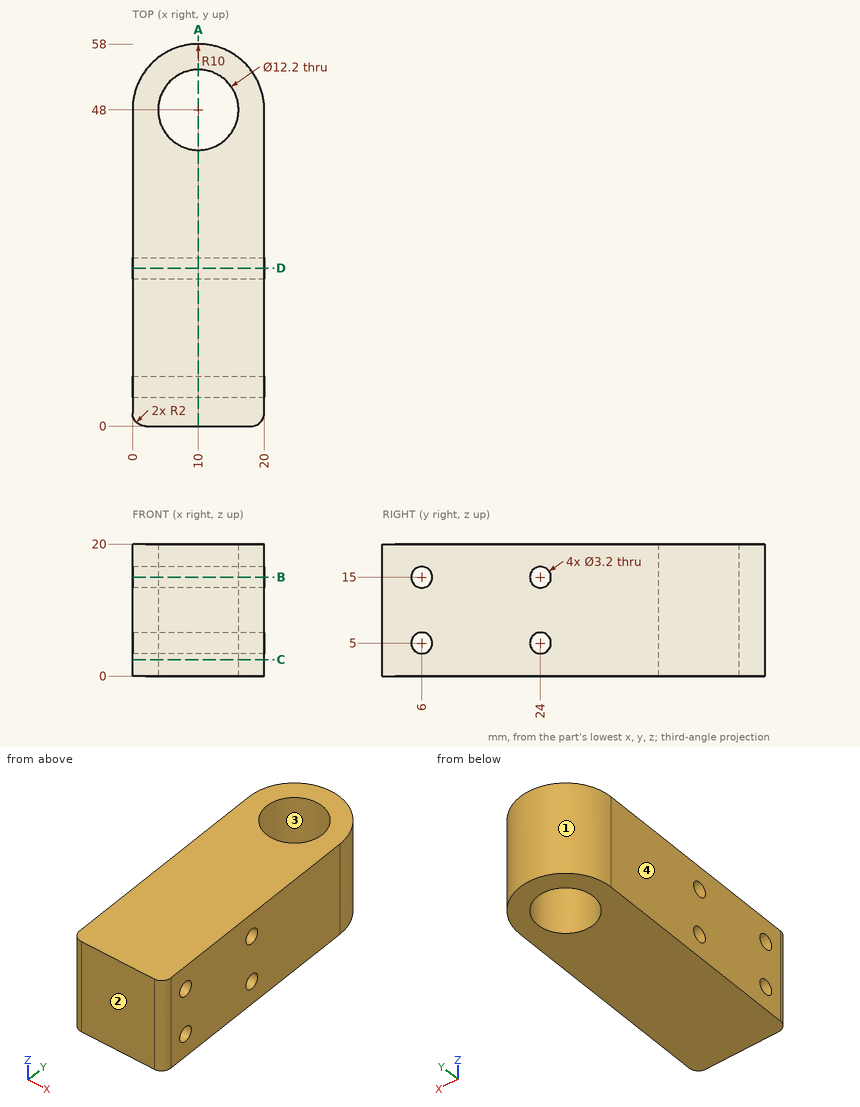
Job drawing, mm, ordinate dimensions from the low corner. One solid piece. Round coordinates to 2 decimals unless told otherwise and drop trailing zeros. Loops run counter-clockwise (first coordinate to the right, second up) from the corner with the lowest first, then second, coordinate; pieces in that order, holes last. Notation, with made-up numbers: M -10,3.5 L 30,3.5 A27 ccw 30,27.5 Z; hole C 50.5,72 d8. An arc over 180 degrees is marked long. Answer as CSV lines item,"result".
1. Flat gauge pins, fed straight in: P1, Ø3.5, axis at y = 6, z = 5, coming from the +X side; P2, Ø10, axis at x = 10, y = 48, coming from the -Z side. Where does each tip first touch, or does it go through?
Resolved:
P1,"stops at x = 20"
P2,"passes through"
2. Cut at A-A on x = 10. Write the cut outline in (y, z), then the cut area to 3 significant figures.
Resolved:
outline,"M 0,0 L 41.9,0 L 41.9,20 L 0,20 Z; M 54.1,0 L 58,0 L 58,20 L 54.1,20 Z; hole C 6,5 d3.2; hole C 6,15 d3.2; hole C 24,5 d3.2; hole C 24,15 d3.2"
area,"884 mm²"
3. Wall check: probe 1 along Y at (x, z) = (9.5, 15); probe 2 along Z at (x, y) = (4.75, 5); probe 3 along Z at (x, y) = (17.5, 6.5). Give the ranges that are in metal, low to high. Write a range as [from, to].
Resolved:
probe 1,"y = [0, 4.4], [7.6, 22.4], [25.6, 41.92], [54.08, 57.99]"
probe 2,"z = [0, 3.75], [6.25, 13.75], [16.25, 20]"
probe 3,"z = [0, 3.48], [6.52, 13.48], [16.52, 20]"
4. Cut at B-B on z = 15. Write the cut outline in (x, y).
Resolved:
outline,"M 0,2 A2 ccw 2,0 L 18,0 A2 ccw 20,2 L 20,4.4 L 0,4.4 Z; M 0,7.6 L 20,7.6 L 20,22.4 L 0,22.4 Z; M 0,25.6 L 20,25.6 L 20,48 A10 ccw 0,48 Z; hole C 10,48 d12.2"
5. Two-plate mould, pull along Y, no slides. Class the marked faces 1, 2, 3 and 4: released by +Y, released by -Y, zero draft, split by the parting line, or undercut.
Resolved:
face 1,"released by +Y"
face 2,"released by -Y"
face 3,"undercut"
face 4,"zero draft"
6. Cut at D-D on y = 24. Write the cut outline in (x, z), then the cut area to 3 significant figures.
Resolved:
outline,"M 0,0 L 20,0 L 20,3.4 L 0,3.4 Z; M 0,6.6 L 20,6.6 L 20,13.4 L 0,13.4 Z; M 0,16.6 L 20,16.6 L 20,20 L 0,20 Z"
area,"272 mm²"
7. Cut at C-C on z = 2.5. Write the cut outline in (x, y), then the cut area to 3 significant figures.
Resolved:
outline,"M 0,2 A2 ccw 2,0 L 18,0 A2 ccw 20,2 L 20,48 A10 ccw 0,48 Z; hole C 10,48 d12.2"
area,"998 mm²"
